Work out the finished part from the listing and answer in its coordinate system (mm). Face numbers are marked on the shaded views. A direction names the side the tool comes from. Round coordinates to 2 decimals unless told otherwise and drop trailing zeros. Order: outer loops, then holes, each group sorted by start corner. A loop starts at its lowest first (then second) coordinate and runs counter-clockwise, first axis right, second up. Notation, with made-up numbers: M 60.25,44 L 84.25,44 A22 cw 84.25,58 Z; hole C 37,-8.75 d3. An arc over 180 degrees is marked long. Return JSON: item names as keys, results as strings.
from build123d import *

# Parameters (mm, degrees)
EXTRUDE_1_DEPTH = 2.5
FILLET_1_R      = 0.5
FILLET_2_R      = 0.5
FILLET_3_R      = 0.5
FILLET_4_R      = 0.5


with BuildPart() as part:
    # 草图1 → 凸台-拉伸1 (new body)
    with BuildSketch(Plane(origin=(0, 0, 0), x_dir=(0, 0, -1), z_dir=(1, 0, 0))):
        Polygon((-5, 1), (5, 1), (5, 2), (12.5, 2), (12.5, -2), (5, -2), (5, -1), (-5, -1), (-5, -2), (-12.5, -2), (-12.5, 2), (-5, 2), align=None)
    extrude(amount=EXTRUDE_1_DEPTH)

    # 圆角1
    fillet_1_edges = [part.edges().sort_by_distance(p)[0] for p in [
        (1.25, 1, -5),
    ]]
    fillet(fillet_1_edges, radius=FILLET_1_R)

    # 圆角2
    fillet_2_edges = [part.edges().sort_by_distance(p)[0] for p in [
        (1.25, -1, -5),
    ]]
    fillet(fillet_2_edges, radius=FILLET_2_R)

    # 圆角3
    fillet_3_edges = [part.edges().sort_by_distance(p)[0] for p in [
        (1.25, 1, 5),
    ]]
    fillet(fillet_3_edges, radius=FILLET_3_R)

    # 圆角4
    fillet_4_edges = [part.edges().sort_by_distance(p)[0] for p in [
        (1.25, -1, 5),
    ]]
    fillet(fillet_4_edges, radius=FILLET_4_R)


solid = part.part
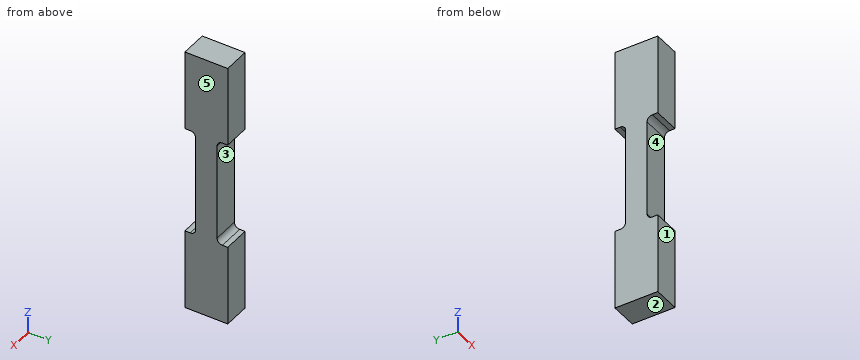
Item 1: Consider line 1 along Z through (x, y) = (0.75, -1.7); line 2 along Y through (x, z) = (1.45, 2.75); line 3 along Z through (x, y) = (2.05, 1.25). Determine where each line is inside the solid, lowest interval first. Write a range as [from, to].
Output:
{"line 1": "z = [-12.5, -5], [5, 12.5]", "line 2": "y = [-1, 1]", "line 3": "z = [-12.5, -4.93], [4.93, 12.5]"}
Item 2: Find section B-B (x = 1.7). Determine the outline of the cut face in (y, z), plus the area to 3 significant figures.
Output:
{"outline": "M -2,-12.5 L 2,-12.5 L 2,-5 L 1.5,-5 A0.5 cw 1,-4.5 L 1,4.5 A0.5 cw 1.5,5 L 2,5 L 2,12.5 L -2,12.5 L -2,5 L -1.5,5 A0.5 cw -1,4.5 L -1,-4.5 A0.5 cw -1.5,-5 L -2,-5 Z", "area": "80.2 mm^2"}
Item 3: Find section A-A (y = -1.75). Determine the outline of the cut face in (x, z).
Output:
{"outline": "M 0,-12.5 L 2.5,-12.5 L 2.5,-5 L 0,-5 Z; M 0,5 L 2.5,5 L 2.5,12.5 L 0,12.5 Z"}
Item 4: Which of the six approach directions +Z, -Z, +X, -X, +Y, -Y give full straight-line access (tool end or side, diameter ignored) to the marked faces 4 and 5?
Output:
{"face 4": "+X, -X, -Y", "face 5": "+Z, -Z, +X, +Y, -Y"}
Item 5: This flat-tipped pin is pushed along its axis until it touches: pin 1 (1.2 mm diameter, centred on x = 2, z = -1.5, fed in from -Y). Where does it stop, or does it pass through?
Output:
{"pin 1": "stops at y = -1"}
Item 6: Find section C-C (z = 1). Determine the outline of the cut face in (x, y).
Output:
{"outline": "M 0,-1 L 2.5,-1 L 2.5,1 L 0,1 Z"}
Item 7: Find section D-D (z = -4.75). Determine the outline of the cut face in (x, y), plus the area to 3 significant figures.
Output:
{"outline": "M 0,-1.07 L 2.5,-1.07 L 2.5,1.07 L 0,1.07 Z", "area": "5.33 mm^2"}
Item 8: The mould has two halves that part along Z. Classify the marked faces 1, 2 and 3: pulls with the +Z half, pulls with the -Z half, needs draft (parallel to the pull), parting line crosses it, or undercut.
Output:
{"face 1": "needs draft", "face 2": "pulls with the -Z half", "face 3": "undercut"}
